Could you check a few things on this model? Use its own coordinates, in mm. Give positions to 0.01 mm unless a question says otherwise; leave off trailing zeros. Write each loop counter-clockwise with the first axis right and the second up, starting at its lowest first coordinate (ties: lowest second). Pieces come first, ordered by that corner, then holes. Notation, with made-up numbers: M 2.5,-32 L 51.5,-32 A28 cw 51.5,-12 Z; hole C -23,-39.5 d6. An arc over 180 degrees is marked long. Use one line per item in the form item = value.
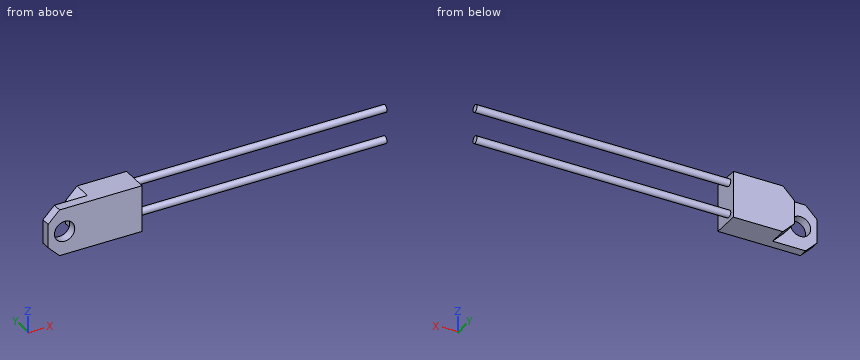
from build123d import *

# Parameters (mm, degrees)
SKETCH1_W           = 18.5
SKETCH1_H           = 9.2
BOSS_EXTRUDE1_DEPTH = 1.8
SKETCH3_W           = 12
SKETCH3_H           = 9.2
BOSS_EXTRUDE3_DEPTH = 3.6
SKETCH2_R           = 0.705
BOSS_EXTRUDE2_DEPTH = 50
SKETCH4_R           = 2
CUT_EXTRUDE1_DEPTH  = 2.8
CHAMFER1_SIZE       = 2.25


with BuildPart() as part:
    # Sketch1 → Boss-Extrude1 (new body)
    with BuildSketch(Plane(origin=(0, 0, 0), x_dir=(1, 0, 0), z_dir=(0, 1, 0))):
        Rectangle(SKETCH1_W, SKETCH1_H)
    extrude(amount=BOSS_EXTRUDE1_DEPTH)

    # Sketch3 → Boss-Extrude3 (add)
    with BuildSketch(Plane(origin=(0, 1.8, 0), x_dir=(1, 0, 0), z_dir=(0, 1, 0))):
        with Locations((3.25, 0)):
            Rectangle(SKETCH3_W, SKETCH3_H)
    extrude(amount=BOSS_EXTRUDE3_DEPTH)

    # Sketch2 → Boss-Extrude2 (add)
    with BuildSketch(Plane(origin=(9.25, 0, 0), x_dir=(0, 0, -1), z_dir=(1, 0, 0))):
        with Locations((-3.15, 3.78)):
            Circle(SKETCH2_R)
        with Locations((3.15, 3.78)):
            Circle(SKETCH2_R)
    extrude(amount=BOSS_EXTRUDE2_DEPTH)

    # Sketch4 → Cut-Extrude1 (cut, through all)
    with BuildSketch(Plane(origin=(0, 1.8, 0), x_dir=(1, 0, 0), z_dir=(0, 1, 0))):
        with Locations((-6, 0)):
            Circle(SKETCH4_R)
    extrude(amount=-CUT_EXTRUDE1_DEPTH, mode=Mode.SUBTRACT)

    # Chamfer1
    chamfer1_edges = [part.edges().sort_by_distance(p)[0] for p in [
        (-9.25, 0.9, -4.6),
        (-9.25, 0.9, 4.6),
        (-2.75, 3.6, -4.6),
        (-2.75, 3.6, 4.6),
    ]]
    chamfer(chamfer1_edges, length=CHAMFER1_SIZE)


solid = part.part
1) I want a section at D-D, the plane z = -3.15. Please give me the cut outline in (x, y) (3 decimals).
Checked values:
outline = M -8.45,0 L 9.25,0 L 9.25,3.075 L 59.25,3.075 L 59.25,4.485 L 9.25,4.485 L 9.25,5.4 L -1.95,5.4 L -1.95,1.8 L -8.45,1.8 Z
2) I want a section at B-B, the plane x = -6. Please give me the cut outline in (y, z).
Checked values:
outline = M 0,-4.6 L 1.8,-4.6 L 1.8,-2 L 0,-2 Z; M 0,2 L 1.8,2 L 1.8,4.6 L 0,4.6 Z
3) I want a section at A-A, the plane z = 0. Please give me the cut outline in (x, y), plus the area to 3 significant figures.
Checked values:
outline = M -9.25,0 L -8,0 L -8,1.8 L -9.25,1.8 Z; M -4,0 L 9.25,0 L 9.25,5.4 L -2.75,5.4 L -2.75,1.8 L -4,1.8 Z
area = 69.3 mm2
4) For pin 1 Ø1.5 at (x, y) = (38, 1.5) entering from +Z; pin 2 Ø3 at (y, z) = (3.5, 0.5) entering from -X; pin 3 Ø1.5 at (y, z) = (2.5, 0) entering from +X; pin 4 Ø1.5 at (x, z) = (35.5, 3) entering from -Y (3 decimals), each with a flat end and sliding along its axis, tell me the tip position at first contact or that it passes through.
Checked values:
pin_1 = through
pin_2 = -2.75
pin_3 = 9.25
pin_4 = 3.075
5) I want a section at C-C, the plane y = 3.78. Please give me the cut outline in (x, z) (3 decimals).
Checked values:
outline = M -2.75,-2.35 L -0.5,-4.6 L 9.25,-4.6 L 9.25,-3.855 L 59.25,-3.855 L 59.25,-2.445 L 9.25,-2.445 L 9.25,2.445 L 59.25,2.445 L 59.25,3.855 L 9.25,3.855 L 9.25,4.6 L -0.5,4.6 L -2.75,2.35 Z
6) If I drill on L1, parallel to X at y = 0.4, z = 0; L2, parallel to Z at x = -6, y = 1.1; L3, parallel to X at y = 3.85, z = 1.75, over which ranges is the centre line in solid material (lowest first)?
Checked values:
L1 = -9.25 to -8, -4 to 9.25
L2 = -4.6 to -2, 2 to 4.6
L3 = -2.75 to 9.25
